The listing builds one solid part. Answer for the finished solid, in the listing's coordinates (mm). A direction names the side the tool comes from. Coordinates: 2 decimals unless noted, no trailing zeros. Order: outer loops, then holes, each group sorted by start corner. A loop starts at its lowest first (then second) coordinate and runs counter-clockwise, first axis right, second up. Notation, with made-up numbers: (28, 80.25) -> (49, 80.25) arc R23 cw to (49, 103.25) -> close; hole circle Ø5 at (-24.5, -11). An arc over 180 degrees is marked (long way). Answer in a Markdown table with one row per item. Add a question column.
```python
from build123d import *

# Parameters (mm, degrees)
F0_W     = 45.72
F0_H     = 45.72
F0_R     = 20.32
F1_DEPTH = 45.72
F2_DEPTH = 71.12
F4_DEPTH = 40.64


with BuildPart() as f1:
    # F0 (on Front) → F1 (new body)
    with BuildSketch(Plane.XZ):
        with Locations((22.86, 22.86)):
            Rectangle(F0_W, F0_H)
        with Locations((22.86, 22.86)):
            Circle(F0_R, mode=Mode.SUBTRACT)
        with Locations((22.86, 22.86)):
            Circle(F0_R)
    extrude(amount=-F1_DEPTH)

    # F0 (on Front) → F2 (join)
    with BuildSketch(Plane.XZ):
        with Locations((22.86, 22.86)):
            Circle(F0_R)
    extrude(amount=F2_DEPTH)

    # F3 (on face) → F4 (join)
    with BuildSketch(Plane(origin=(0, 45.72, 0), x_dir=(-1, 0, 0), z_dir=(0, 1, 0))):
        Polygon((-16.51, 19.193826), (-16.51, 26.526174), (-22.86, 30.192348), (-29.21, 26.526174), (-29.21, 19.193826), (-22.86, 15.527652), align=None)
    extrude(amount=F4_DEPTH)


solid = f1.part
```
Q1. A cutting plane is placed at D-D (z = 13.5). Determine the outline of the cut face in (x, y), then the cut area to 3 significant figures.
Q2. Straight lines are drawn through the part: line 1 (X direction, y = -21.5, z = 24); line 2 (Y direction, x = 12, z = 16.5); line 3 (Y direction, x = 7.5, z = 41.5). For each, find the intervals that lie inside material, in ascending order.
Q3. A cutting plane is placed at A-A (y = 73.5). Determine the outline of the cut face in (x, z), then the cut area to 3 significant figures.
Q4. Given pin 1 (8 mm diameter, centred on y = 65.5, z = 24.5, fed in from +X); pin 2 (8 mm diameter, centred on x = 35.5, y = 50.5, fed in from +Z); pin 3 (4 mm diameter, centred on x = 22, y = -41.5, fed in from +Z); pin 4 (3 mm diameter, centred on y = -41, z = 26, fed in from +X), each flat-ended and moving along its own axis, determine where each tip first touches the part or whether it passes through.
Q5. For faces 1 (the face through (25.991, 65.756, 28.385)), 2 (the face through (26.1, 65.8, 17.4)), 3 (the face through (28, 45.72, 18)), 4 (the face through (19.729, 65.756, 17.335)), 5 (the face through (2, 0, 23)), determine the directions among +Z, -Z, +X, -X, +Y, -Y from which every point of the face is accessible in a straight line to the end or side of a thin tool.
Q6. A cutting plane is placed at C-C (x = 9.5). Determine the outline of the cut face in (y, z), then the cut area to 3 significant figures.
Q7. A cutting plane is placed at B-B (z = 22.86). Determine the outline of the cut face in (x, y).
Returned:
| question | item | result |
|---|---|---|
| 1 | outline | (0, 0) -> (4.82, 0) -> (4.82, -71.12) -> (40.9, -71.12) -> (40.9, 0) -> (45.72, 0) -> (45.72, 45.72) -> (0, 45.72) -> close |
| 1 | area | 4,660 mm² |
| 2 | line 1 | x = 2.57 to 43.15 |
| 2 | line 2 | y = -71.12 to 45.72 |
| 2 | line 3 | y = 0 to 45.72 |
| 3 | outline | (16.51, 19.19) -> (22.86, 15.53) -> (29.21, 19.19) -> (29.21, 26.53) -> (22.86, 30.19) -> (16.51, 26.53) -> close |
| 3 | area | 140 mm² |
| 4 | pin 1 | stops at x = 29.21 |
| 4 | pin 2 | passes through |
| 4 | pin 3 | stops at z = 43.18 |
| 4 | pin 4 | stops at x = 43.11 |
| 5 | face 1 | +Z, +X, +Y |
| 5 | face 2 | -Z, +X, +Y |
| 5 | face 3 | +Y |
| 5 | face 4 | -Z, -X, +Y |
| 5 | face 5 | -Y |
| 6 | outline | (-71.12, 7.55) -> (0, 7.55) -> (0, 0) -> (45.72, 0) -> (45.72, 45.72) -> (0, 45.72) -> (0, 38.17) -> (-71.12, 38.17) -> close |
| 6 | area | 4,270 mm² |
| 7 | outline | (0, 0) -> (2.54, 0) -> (2.54, -71.12) -> (43.18, -71.12) -> (43.18, 0) -> (45.72, 0) -> (45.72, 45.72) -> (29.21, 45.72) -> (29.21, 86.36) -> (16.51, 86.36) -> (16.51, 45.72) -> (0, 45.72) -> close |
